Autodesk Inventor part; units mm, degrees
ref_plane "YZ Plane" through (0, 0, 0) normal (1, 0, 0) x (0, 1, 0)
ref_plane "XZ Plane" through (0, 0, 0) normal (0, 1, 0) x (-1, 0, 0)
ref_plane "XY Plane" through (0, 0, 0) normal (0, 0, 1) x (1, 0, 0)
sketch "Sketch1" plane through (0, 0, 0) normal (0, 1, 0) x (-1, 0, 0)
  circle A0 centre (0, 0) radius 8.255
  line L0 (-6.5405, -3.7762) -> (-6.5405, 3.7762)
  line L1 (-6.5405, 3.7762) -> (0, 7.5523)
  line L2 (0, 7.5523) -> (6.5405, 3.7762)
  line L3 (6.5405, 3.7762) -> (6.5405, -3.7762)
  line L4 (6.5405, -3.7762) -> (0, -7.5523)
  line L5 (0, -7.5523) -> (-6.5405, -3.7762)
  dimension "d0" = 16.51
  dimension "d1" = 13.081
extrude "Extrusion1" add sketch "Sketch1" along normal blind 12.7
properties part number "S1"
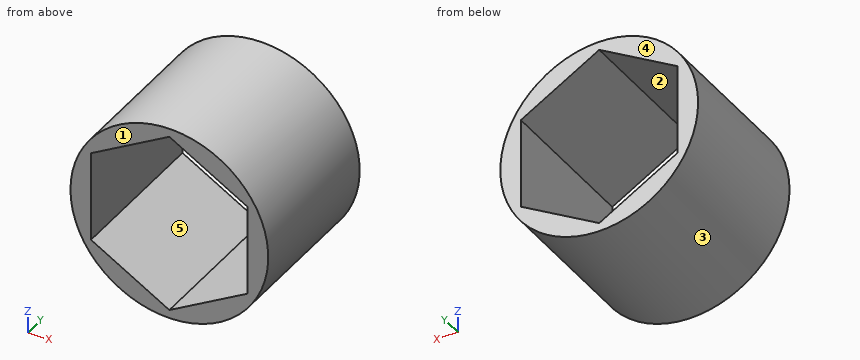
Design review of the part built by this model. Coordinates are the model's own, in mm. Face numbers are marked on the shaded views. A direction names the side the tool comes from. Coordinates: 2 decimals unless noted, no trailing zeros. Order: outer loops, then holes, each group sorted by start corner. A loop starts at its lowest first (then second) coordinate and runs counter-clockwise, first axis right, second up. Notation, with made-up numbers: (18, 21.25) - (45, 21.25) arc R25 ccw to (45, 40.25) - close; hole circle Ø3 at (77.5, -2). An arc over 180 degrees is marked (long way). One line per question, with ' | ' between items.
Q1. Consider section C-C, the plane y = 12. Give the boundary of the cut face in (x, z) (1 decimal).
Answer key:
outline: circle Ø16.5 at (0, 0); hole (-6.5, -3.8) - (0, -7.6) - (6.5, -3.8) - (6.5, 3.8) - (0, 7.6) - (-6.5, 3.8) - close
Q2. Consider section A-A, the plane z = 0. Give the boundary of the cut face in (x, y) (1 decimal), then the cut area to 3 significant figures.
Answer key:
outline: (-8.3, 0) - (-6.5, 0) - (-6.5, 12.7) - (-8.3, 12.7) - close; (6.5, 0) - (8.3, 0) - (8.3, 12.7) - (6.5, 12.7) - close | area: 43.5 mm2
Q3. The part is to be moulded in two halves that separate along X. For the marked faces 3, 4 and 5, say which applies: +X half, -X half, draft (parallel to the pull), parting line (faces both ways), or undercut.
Answer key:
face 3: parting line | face 4: draft | face 5: undercut
Q4. Clearance check with flat-ended pins moving along their axes: pin 1 Ø3 at (x, y) = (4.5, 11) entering from -Z; pin 2 Ø3 at (y, z) = (3.5, 5) entering from -X; pin 3 Ø2.5 at (y, z) = (5, 1.5) entering from -X. State where each tip first meets the part, or that it passes through.
Answer key:
pin 1: stops at z = -7.69 | pin 2: stops at x = -7.48 | pin 3: stops at x = -8.25
Q5. Consider section B-B, the plane x = -3. Give the boundary of the cut face in (y, z), then the cut area to 3 significant figures.
Answer key:
outline: (0, -7.69) - (12.7, -7.69) - (12.7, -5.82) - (0, -5.82) - close; (0, 5.82) - (12.7, 5.82) - (12.7, 7.69) - (0, 7.69) - close | area: 47.5 mm2
Q6. For the marked faces 1 and 2, list the 3-axis set-ups (+Z, -Z, +X, -X, +Y, -Y) from which the entire face can be reached by the end or side of a thin tool; tool diameter is ignored.
Answer key:
face 1: +Z, -Z, +X, -X, -Y | face 2: +Y, -Y
Q7. To check wall thickness, follow line 1 along X through (y, z) = (3.75, 3.5); line 2 along X through (y, z) = (6, -6); line 3 along Z through (x, y) = (-6.5, 2.25). State the ranges of each line that lie inside material, in increasing order.
Answer key:
line 1: x = -7.48 to -6.54, 6.54 to 7.48 | line 2: x = -5.67 to -2.69, 2.69 to 5.67 | line 3: z = -5.09 to -3.8, 3.8 to 5.09
